```python
from build123d import *

# Parameters (mm, degrees)
SKETCH1_RX          = 101.6
SKETCH1_RY          = 63.5
SKETCH1_R           = 19.05
BOSS_EXTRUDE1_DEPTH = 3.175


with BuildPart() as part:
    # Sketch1 → Boss-Extrude1 (new body)
    with BuildSketch(Plane(origin=(0, 0, 0), x_dir=(1, 0, 0), z_dir=(0, 1, 0))):
        with Locations(Location((0, 0), (0, 0, 180))):
            Ellipse(SKETCH1_RX, SKETCH1_RY)
        with Locations(Location((0, 0, 0), (0, 0, 270))):
            Circle(SKETCH1_R, mode=Mode.SUBTRACT)
        Polygon((-61.535303163, 0), (-68.867651581, 12.7), (-83.532348419, 12.7), (-90.864696837, 0), (-83.532348419, -12.7), (-68.867651581, -12.7), align=None, mode=Mode.SUBTRACT)
        Polygon((90.864696837, 0), (83.532348419, 12.7), (68.867651581, 12.7), (61.535303163, 0), (68.867651581, -12.7), (83.532348419, -12.7), align=None, mode=Mode.SUBTRACT)
        with BuildLine():
            Line((50.8, -19.05), (50.8, -12.7))
            ThreePointArc((50.8, -12.7), (44.45, -6.35), (38.1, -12.7))
            Line((38.1, -12.7), (38.1, -19.05))
            ThreePointArc((38.1, -19.05), (34.380256121, -28.030256121), (25.4, -31.75))
            Line((25.4, -31.75), (19.05, -31.75))
            ThreePointArc((19.05, -31.75), (12.7, -38.1), (19.05, -44.45))
            Line((19.05, -44.45), (25.4, -44.45))
            ThreePointArc((25.4, -44.45), (43.360512242, -37.010512242), (50.8, -19.05))
        make_face(mode=Mode.SUBTRACT)
        with BuildLine():
            Line((-25.4, -31.75), (-19.05, -31.75))
            ThreePointArc((-19.05, -31.75), (-12.7, -38.1), (-19.05, -44.45))
            Line((-19.05, -44.45), (-25.4, -44.45))
            ThreePointArc((-25.4, -44.45), (-43.360512242, -37.010512242), (-50.8, -19.05))
            Line((-50.8, -19.05), (-50.8, -12.7))
            ThreePointArc((-50.8, -12.7), (-44.45, -6.35), (-38.1, -12.7))
            Line((-38.1, -12.7), (-38.1, -19.05))
            ThreePointArc((-38.1, -19.05), (-34.380256121, -28.030256121), (-25.4, -31.75))
        make_face(mode=Mode.SUBTRACT)
        with BuildLine():
            Line((25.4, 31.75), (19.05, 31.75))
            ThreePointArc((19.05, 31.75), (12.7, 38.1), (19.05, 44.45))
            Line((19.05, 44.45), (25.4, 44.45))
            ThreePointArc((25.4, 44.45), (43.360512242, 37.010512242), (50.8, 19.05))
            Line((50.8, 19.05), (50.8, 12.7))
            ThreePointArc((50.8, 12.7), (44.45, 6.35), (38.1, 12.7))
            Line((38.1, 12.7), (38.1, 19.05))
            ThreePointArc((38.1, 19.05), (34.380256121, 28.030256121), (25.4, 31.75))
        make_face(mode=Mode.SUBTRACT)
        with BuildLine():
            Line((-25.4, 31.75), (-19.05, 31.75))
            ThreePointArc((-19.05, 31.75), (-12.7, 38.1), (-19.05, 44.45))
            Line((-19.05, 44.45), (-25.4, 44.45))
            ThreePointArc((-25.4, 44.45), (-43.360512242, 37.010512242), (-50.8, 19.05))
            Line((-50.8, 19.05), (-50.8, 12.7))
            ThreePointArc((-50.8, 12.7), (-44.45, 6.35), (-38.1, 12.7))
            Line((-38.1, 12.7), (-38.1, 19.05))
            ThreePointArc((-38.1, 19.05), (-34.380256121, 28.030256121), (-25.4, 31.75))
        make_face(mode=Mode.SUBTRACT)
    extrude(amount=BOSS_EXTRUDE1_DEPTH)


solid = part.part
```
Design review of the part built by this model. Coordinates are the model's own, in mm. Give positions to 0.01 mm unless a question says otherwise; leave off trailing zeros. Return JSON: item names as keys, results as strings. Group by question number.
(1) Mouldability with a two-part tool opening along Z and no side actions: class faces 1 (the flat face through (-21, 0, 1)), 2 (the cylindrical face through (12.7, 1.6, 38)), 3 (the cylindrical face through (43.16, 1.57, -37.21)) as +Z half, -Z half, draft (parallel to the pull), parting line (faces both ways), or undercut.
(2) We need section A-A, the plane x = -44.45. Give the number of separate pieces and of enclosed holes in the cut face, then the cut area to 3 significant figures.
(3) Insertion check: pin 1 (1.6 mm diameter, centred on y = 1.5, z = -14.5, fed in from +X); pin 2 (1 mm diameter, centred on y = 1, z = 44.5, fed in from -X); pin 3 (1 mm diameter, centred on x = 10, y = 2, fed in from -Z). Each pin has a flat end and moves straight along its axis. Give the tip position at first contact, or say it passes through.
(4) To check wall thickness, follow probe 1 along X at (y, z) = (1.3, 0); probe 2 along Z at (x, y) = (36.5, 3); probe 3 along Z at (x, y) = (-24, 1.85). State the ranges of each line that lie inside material, in increasing order.
Reported:
{
 "1": {"face 1": "draft", "face 2": "undercut", "face 3": "undercut"},
 "2": {"separate pieces": "3", "enclosed holes": "0", "area": "175 mm2"},
 "3": {"pin 1": "stops at x = 99.21", "pin 2": "stops at x = -73.26", "pin 3": "stops at z = -63.22"},
 "4": {"probe 1": "x = -101.6 to -90.86, -61.54 to -19.05, 19.05 to 61.54, 90.86 to 101.6", "probe 2": "z = -59.26 to -41.9, -25.22 to 25.22, 41.9 to 59.26", "probe 3": "z = -61.7 to -44.45, -31.75 to 31.75, 44.45 to 61.7"}
}
